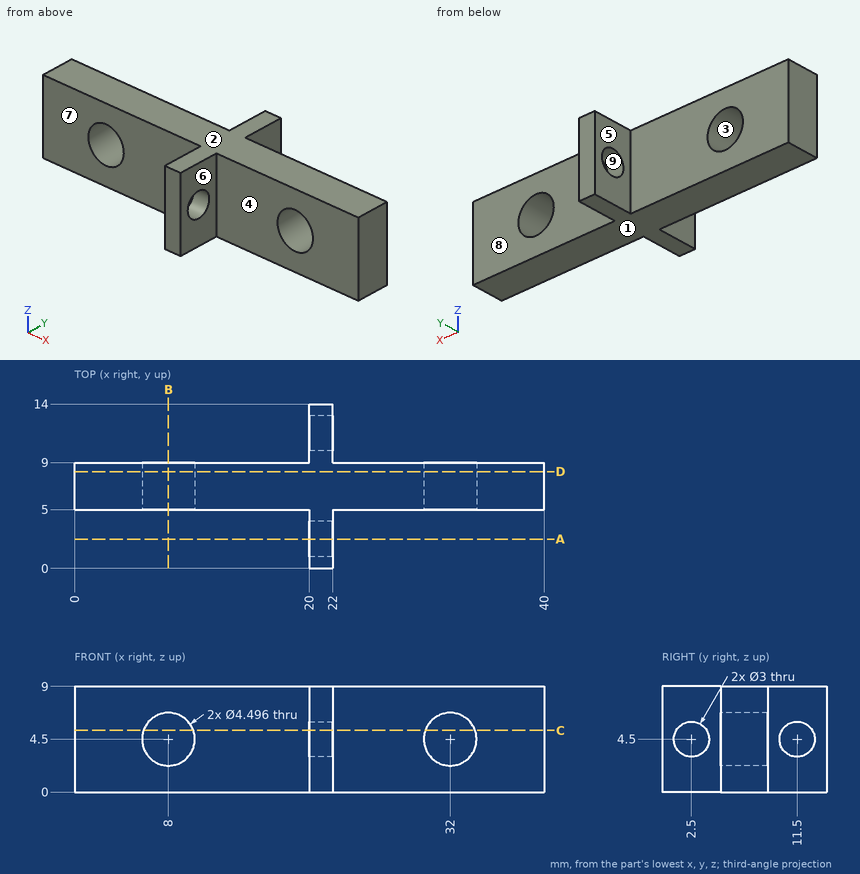
Geometry check sheet. Reference: drawing and pictorial views, mm from the part's lowest x, y, z. A direction names the side the tool comes from. Give positions to 0.01 mm unless a question says otherwise; leave off trailing zeros. Loops run counter-clockwise (first coordinate to the right, second up) from the corner with the lowest first, then second, coordinate; pieces in that order, holes last.
1. Section check C-C, the plane z = 5.25. Enter the section's corners in (x, y), then the cut area to 3 significant figures.
2. Set-up check for the marked faces 5, 6, 7, 8 and 9: record each of +Z, -Z, +X, -X, +Y, -Y from which the full face is reachable in a straight line by a thin tool's end or side.
3. Thickness scan on line 1 (X direction, y = 7.3, z = 4.5); line 2 (Y direction, x = 20.65, z = 4.5); line 3 (Y direction, x = 6, z = 1.5). Record the ranges inside material, lowest first.
4. Mould release check, pull along Z, two halves, no side actions. Record for the marked faces 1, 2, 3 and 4: released by +Z, released by -Z, zero draft, split by the parting line, or undercut.
5. Section check A-A, the plane y = 2.5. Enter the section's corners in (x, z).
6. Go/stop test with flat-tipped pins: pin 1 Ø1.5 at (y, z) = (10.5, 2.5) entering from -X; pin 2 Ø4 at (x, z) = (32, 4.5) entering from -Y; pin 3 Ø2.5 at (x, z) = (28.5, 6.5) entering from +Y; pin 4 Ø2.5 at (x, z) = (9.5, 4.5) entering from -Y. Record where each tip stops, or that it passes through.
7. Section check B-B, the plane x = 8. Enter the section's corners in (y, z), then the cut area to 3 significant figures.
8. Section check D-D, the plane y = 8.25. Enter the section's corners in (x, z), then the cut area to 3 significant figures.
Geometry says:
1. outline: (0, 5) - (5.88, 5) - (5.88, 9) - (0, 9) - close; (10.12, 5) - (20, 5) - (20, 3.8) - (22, 3.8) - (22, 5) - (29.88, 5) - (29.88, 9) - (22, 9) - (22, 10.2) - (20, 10.2) - (20, 9) - (10.12, 9) - close; (20, 0) - (22, 0) - (22, 1.2) - (20, 1.2) - close; (20, 12.8) - (22, 12.8) - (22, 14) - (20, 14) - close; (34.12, 5) - (40, 5) - (40, 9) - (34.12, 9) - close
1. area: 136 mm2
2. face 5: +Z, -Z, -X, +Y
2. face 6: +Z, -Z, +X, -Y
2. face 7: +Z, -Z, -X, -Y
2. face 8: +Z, -Z, +X, +Y
2. face 9: +X, -X
3. line 1: x = 0 to 5.75, 10.25 to 29.75, 34.25 to 40
3. line 2: y = 0 to 1, 4 to 10, 13 to 14
3. line 3: y = 5 to 9
4. face 1: released by -Z
4. face 2: released by +Z
4. face 3: undercut
4. face 4: zero draft
5. outline: (20, 0) - (22, 0) - (22, 3) - (20, 3) - close; (20, 6) - (22, 6) - (22, 9) - (20, 9) - close
6. pin 1: stops at x = 20
6. pin 2: passes through
6. pin 3: stops at y = 9
6. pin 4: stops at y = 5
7. outline: (5, 0) - (9, 0) - (9, 2.25) - (5, 2.25) - close; (5, 6.75) - (9, 6.75) - (9, 9) - (5, 9) - close
7. area: 18.0 mm2
8. outline: (0, 0) - (40, 0) - (40, 9) - (0, 9) - close; hole circle Ø4.5 at (8, 4.5); hole circle Ø4.5 at (32, 4.5)
8. area: 328 mm2
